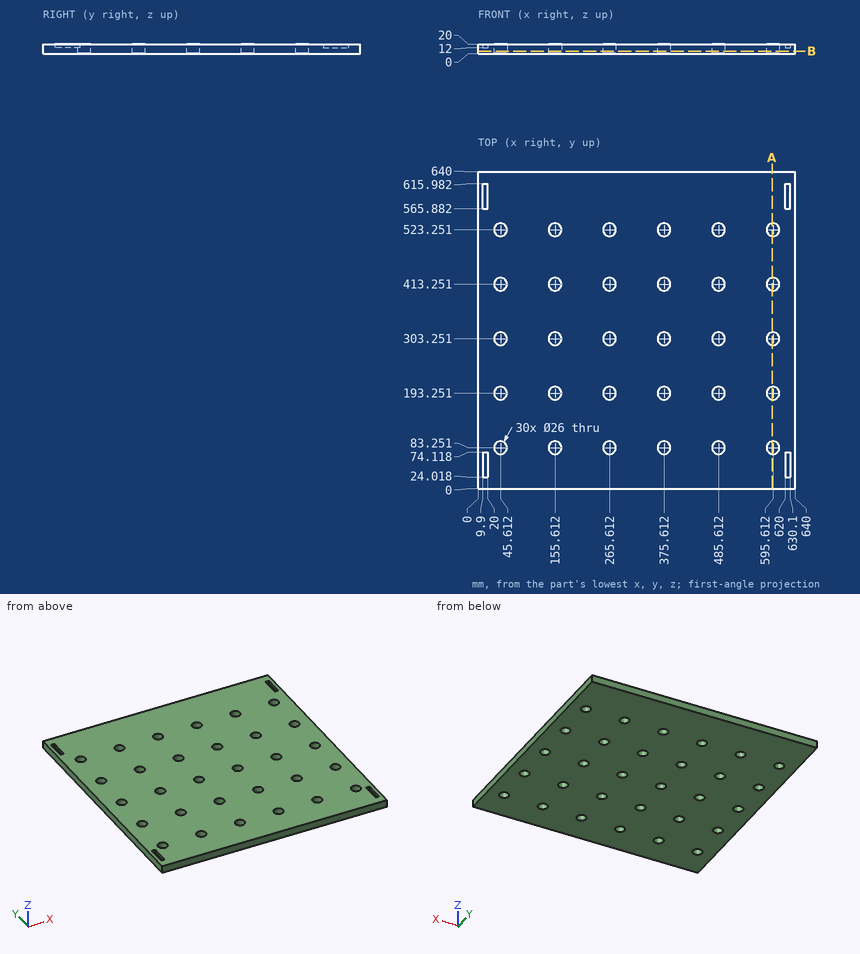
For this review, use the dimensioned drawing (mm, ordinates from the lowest corner) and the shaded views. Give positions to 0.01 mm unless a question says otherwise; leave off trailing zeros. Loops run counter-clockwise (first coordinate to the right, second up) from the corner with the lowest first, then second, coordinate; pieces in that order, holes last.
Item 1: For line 1 along Y through (x, z) = (376.5, 5.5); line 2 along X through (y, z) = (593.5, 18.25); line 3 along Y through (x, z) = (153, 7) (1 decimal), list the stretches that pass through material, from the lowest coordinate up.
Item 2: Take a section at B-B, the plane z = 5.75. Give the number of separate pieces and of enclosed holes in the cut face, and give its area (3 significant figures).
Item 3: Take a section at A-A, the plane x = 594. State the section outline as (y, z) points.
Calculated:
1. line 1: y = 0 to 70.28, 96.22 to 180.28, 206.22 to 290.28, 316.22 to 400.28, 426.22 to 510.28, 536.22 to 640
1. line 2: x = 0 to 9.9, 20 to 620, 630.1 to 640
1. line 3: y = 0 to 70.5, 96 to 180.5, 206 to 290.5, 316 to 400.5, 426 to 510.5, 536 to 640
2. separate pieces: 1
2. enclosed holes: 30
2. area: 394,000 mm2
3. outline: (0, 0) - (70.35, 0) - (70.35, 20) - (0, 20) - close; (96.15, 0) - (180.35, 0) - (180.35, 20) - (96.15, 20) - close; (206.15, 0) - (290.35, 0) - (290.35, 20) - (206.15, 20) - close; (316.15, 0) - (400.35, 0) - (400.35, 20) - (316.15, 20) - close; (426.15, 0) - (510.35, 0) - (510.35, 20) - (426.15, 20) - close; (536.15, 0) - (640, 0) - (640, 20) - (536.15, 20) - close
